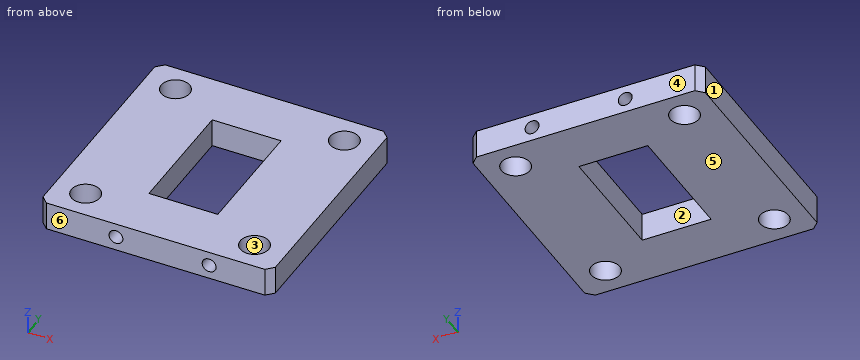
Autodesk Inventor part; units mm, degrees
ref_plane "YZ Plane" through (0, 0, 0) normal (1, 0, 0) x (0, 1, 0)
ref_plane "XZ Plane" through (0, 0, 0) normal (0, 1, 0) x (-1, 0, 0)
ref_plane "XY Plane" through (0, 0, 0) normal (0, 0, 1) x (1, 0, 0)
sketch "Sketch3" plane through (0, 0, 0) normal (0, 0, 1) x (1, 0, 0)
  line L0 (-15.7, -16.7) -> (15.7, -16.7)
  line L1 (16.7, -15.7) -> (16.7, 15.7)
  line L2 (15.7, 16.7) -> (-15.7, 16.7)
  line L3 (-16.7, 15.7) -> (-16.7, -15.7)
  line L4 (-16.7, -16.7) -> (16.7, 16.7) construction
  line L5 (16.7, -16.7) -> (-16.7, 16.7) construction
  line L6 (-15.7, 16.7) -> (-16.7, 15.7)
  line L7 (15.7, 16.7) -> (16.7, 15.7)
  line L8 (16.7, -15.7) -> (15.7, -16.7)
  line L9 (-16.7, -15.7) -> (-15.7, -16.7)
  line L10 (-4.9497, -8.8994) -> (4.9497, -8.8994)
  line L11 (4.9497, -8.8994) -> (4.9497, 8.8994)
  line L12 (4.9497, 8.8994) -> (-4.9497, 8.8994)
  line L13 (-4.9497, 8.8994) -> (-4.9497, -8.8994)
  line L14 (-4.9497, -8.8994) -> (4.9497, 8.8994) construction
  line L15 (4.9497, -8.8994) -> (-4.9497, 8.8994) construction
  circle A0 centre (-12.14, 12.625) radius 2.045
  circle A1 centre (12.14, 12.625) radius 2.045
  line L16 (0, -16.7) -> (0, 16.7) construction
  circle A2 centre (-12.14, -12.625) radius 2.045
  circle A3 centre (12.14, -12.625) radius 2.045
  line L17 (12.14, 12.625) -> (-12.14, 12.625) construction
  line L18 (-12.14, 12.625) -> (-12.14, -12.625) construction
  line L19 (-12.14, -12.625) -> (12.14, -12.625) construction
  line L20 (12.14, -12.625) -> (12.14, 12.625) construction
  line L21 (-16.7, 0) -> (16.7, 0) construction
  point P0 (0, 0)
  point P1 (0, 0)
  dimension "d0" = 33.4
  dimension "d1" = 33.4
  dimension "d2" = 1
  dimension "d3" = 1
  dimension "d4" = 1
  dimension "d5" = 1
  dimension "d6" = 1
  dimension "d7" = 1
  dimension "d8" = 1
  dimension "d9" = 1
  dimension "d10" = 9.8994
  dimension "d11" = 17.7988
  dimension "d12" = 4.09
  dimension "d13" = 4.09
  dimension "d17" = 4.09
  dimension "d19" = 24.28
  dimension "d20" = 25.25
  dimension "d21" = 4.09
  dimension "d22" = 12.625
  dimension "d23" = 12.14
extrude "Extrusion1" add sketch "Sketch3" along normal blind 4.1
sketch "Sketch6" plane through (-15.7, 16.7, 0) normal (0, 1, 0) x (1, 0, 0)
  circle A0 centre (10, -2.05) radius 1
  circle A1 centre (23.4, -2.05) radius 1
  line L0 (-1, 0) -> (-1, -4.1)
  line L1 (32.4, 0) -> (32.4, -4.1)
  line L2 (31.4, 0) -> (0, 0)
  line L3 (31.4, -4.1) -> (0, -4.1)
  point P0 (15.7, 0)
  dimension "d54" = 2
  dimension "d55" = 2
  dimension "d57" = 9
  dimension "d58" = 13.4
  dimension "d59" = 2.05
  dimension "d60" = 2.05
sketch "Sketch7" plane through (-15.7, -16.7, 0) normal (0, -1, 0) x (1, 0, 0)
  circle A0 centre (23.4, 2.05) radius 1
  circle A1 centre (10, 2.05) radius 1
  line L0 (0, 0) -> (31.4, 0)
  line L1 (0, 4.1) -> (31.4, 4.1)
  line L2 (32.4, 0) -> (32.4, 4.1)
  line L3 (-1, 0) -> (-1, 4.1)
  point P0 (15.7, 0)
  dimension "d61" = 2
  dimension "d62" = 2
  dimension "d63" = 2.05
  dimension "d64" = 2.05
  dimension "d65" = 2.05
  dimension "d67" = 11
  dimension "d81" = 13.4
extrude "Extrusion4" cut sketch "Sketch7" against normal blind 8
extrude "Extrusion5" cut sketch "Sketch6" against normal blind 7
thread "Thread5"
thread "Thread6"
thread "Thread7"
thread "Thread8"
equation "\"d3\" = d2"
equation "\"d5\" = d4"
equation "\"d6\" = d4"
equation "\"d7\" = d6"
equation "\"d8\" = d4"
equation "\"d9\" = d8"
properties part number "WG18FLANGE" material "Brass, Soft Yellow"
Input: part model. Units: mm. Frame: model coordinates. Face numbers are marked on the shaded views. A direction names the side the tool comes from. Round coordinates to 2 decimals unless told otherwise and drop trailing zeros. Loops run counter-clockwise (first coordinate to the right, second up) from the corner with the lowest first, then second, coordinate; pieces in that order, holes last. Notation, with made-up numbers: (-27, 9) -> (19, 9) arc R36 cw to (19, 48) -> close; hole circle Ø5 at (73, -23.5). An arc over 180 degrees is marked (long way). Write each question's results on one line, items separated by ' | '.
1. First-contact query: P1, Ø3.5, axis at x = -12.14, y = 12.625, coming from the +Z side; P2, Ø1.6, axis at x = 7.7, z = 2.05, coming from the +Y side; P3, Ø1.2, axis at x = -5.7, z = 2.05, coming from the -Y side. Flat tips, straight axial feed; report the tip coordinate or a pass-through.
Geometry results:
P1: through | P2: y = 9.7 | P3: y = -8.7
2. Ray query, line 1 (X direction, y = -3.5, z = 2.7); line 2 (Z direction, x = 7.7, y = -12.75); line 3 (Y direction, x = 12, z = 0.55). Return the intervals inside material, ascending. Write a range as from..to.
Geometry results:
line 1: -16.7..-4.95, 4.95..16.7 | line 2: 0..1.05, 3.05..4.1 | line 3: -16.7..-14.67, -10.58..10.58, 14.67..16.7
3. Section C-C (z = 2.05). State how many separate pieces and enclosed holes the cut face has, and give its area (3 significant figures).
Geometry results:
separate pieces: 1 | enclosed holes: 4 | area: 825 mm2
4. Set-up query: the marked faces 1 and 2. Return all of +Z, -Z, +X, -X, +Y, -Y with unobstructed straight access to the full face (end or side cutting, diameter ignored); none if empty.
Geometry results:
face 1: +Z, -Z, -X, +Y, -Y | face 2: +Z, -Z
5. Mould query, pull axis Y, two halves, no side actions, for the marked faces 3, 4, 5 and 6. Classes: +Y half, -Y half, draft (parallel to the pull), parting line (faces both ways), or undercut.
Geometry results:
face 3: undercut | face 4: +Y half | face 5: draft | face 6: -Y half
6. Section B-B (y = 8.5). Return loops of the section in (x, z).
Geometry results:
outline: (-16.7, 0) -> (-4.95, 0) -> (-4.95, 4.1) -> (-16.7, 4.1) -> close; (4.95, 0) -> (16.7, 0) -> (16.7, 4.1) -> (4.95, 4.1) -> close
7. Section A-A (x = -12.14). Return loops of the section in (y, z), and give its area (3 significant figures).
Geometry results:
outline: (-16.7, 0) -> (-14.67, 0) -> (-14.67, 4.1) -> (-16.7, 4.1) -> close; (-10.58, 0) -> (10.58, 0) -> (10.58, 4.1) -> (-10.58, 4.1) -> close; (14.67, 0) -> (16.7, 0) -> (16.7, 4.1) -> (14.67, 4.1) -> close | area: 103 mm2
8. Section D-D (x = 7.7). Return loops of the section in (y, z).
Geometry results:
outline: (-16.7, 0) -> (16.7, 0) -> (16.7, 1.05) -> (9.7, 1.05) -> (9.7, 3.05) -> (16.7, 3.05) -> (16.7, 4.1) -> (-16.7, 4.1) -> (-16.7, 3.05) -> (-8.7, 3.05) -> (-8.7, 1.05) -> (-16.7, 1.05) -> close
